Verification items for this drawing (mm, ordinates from the low corner). Round coordinates to 2 decimals unless told otherwise and drop trailing zeros. Loops run counter-clockwise (first coordinate to the right, second up) from the corner with the lowest first, then second, coordinate; pieces in that order, holes last. Notation, with made-up numbers: M 42,32 L 86,32 A11 ccw 86,44 Z; hole C 7,2.25 d9. An arc over 180 degrees is marked long. Write item = value, one per line. Start each with the question number.
(1) Scan lines: L1, parallel to Z at x = 2.9, y = 3.25; L2, parallel to Z at x = 3.3, y = 5.5; L3, parallel to X at y = 12.75, z = 2.8. Record each from-to range of solid material in increasing order. Write a range as from..to.
(2) Cross-section at D-D on x = 1.2. Record the boundary of the cut face in (y, z).
(3) Mould release check, pull along Z, two halves, no side actions. Record for the marked faces 1, 2, 3 and 4: pulls with the +Z half, pulls with the -Z half, needs draft (parallel to the pull), parting line crosses it, or undercut.
(4) Go/stop test with a flat-tipped pin: P1, Ø3, axis at y = 7.5, z = 3.5, coming from the -X side. Record where the tip stops, or that it passes through.
(5) Cross-section at A-A on x = 3.2. Record the boundary of the cut face in (y, z).
(6) Cross-section at B-B on z = 2.25. Record the boundary of the cut face in (x, y) (1 decimal).
(7) Cross-section at C-C on y = 6. Record the boundary of the cut face in (x, z).
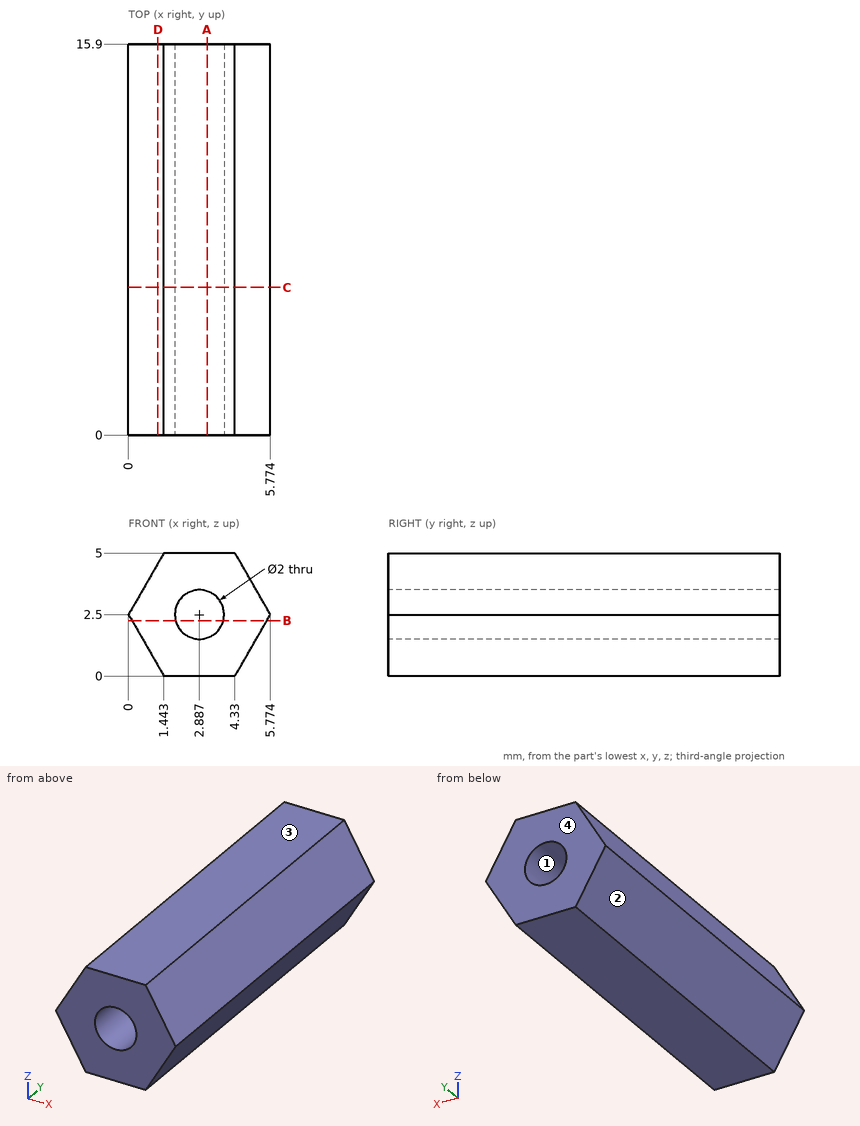
Result:
q1.L1 = 0..1.5, 3.5..5
q1.L2 = 0..1.59, 3.41..5
q1.L3 = 0.17..1.93, 3.84..5.6
q2.outline = M 0,0.42 L 15.9,0.42 L 15.9,4.58 L 0,4.58 Z
q3.face_1 = undercut
q3.face_2 = pulls with the -Z half
q3.face_3 = pulls with the +Z half
q3.face_4 = needs draft
q4.P1 = 0
q5.outline = M 0,0 L 15.9,0 L 15.9,1.55 L 0,1.55 Z; M 0,3.45 L 15.9,3.45 L 15.9,5 L 0,5 Z
q6.outline = M 0.1,0 L 1.9,0 L 1.9,15.9 L 0.1,15.9 Z; M 3.9,0 L 5.6,0 L 5.6,15.9 L 3.9,15.9 Z
q7.outline = M 0,2.5 L 1.44,0 L 4.33,0 L 5.77,2.5 L 4.33,5 L 1.44,5 Z; hole C 2.89,2.5 d2
